from build123d import *

# Parameters (mm, degrees)
F1_DEPTH  = 46
F2_R      = 1
F3_DEPTH  = 1.5
F5_DEPTH  = 40
F6_R      = 1.5
F7_DEPTH  = 1.5
F8_R      = 10
F9_DEPTH  = 1.5
F10_DEPTH = 1.259
F11_DEPTH = 1.259


with BuildPart() as f1:
    # F0 (on Top) → F1 (new body)
    with BuildSketch(Plane.XY):
        Polygon((-20, 74.7819926235), (-21.5, 74.7819926235), (-21.5, 16.0825311363), (-1.5, -0.6994614872), (-1.5, -10), (0, -10), (0, 0), (-20, 16.7819926235), align=None)
    extrude(amount=F1_DEPTH)

    # F2 (on face) → F3 (cut, through all)
    with BuildSketch(Plane(origin=(-1.5, 0, 0), x_dir=(0, -1, 0), z_dir=(-1, 0, 0))):
        with Locations((6, 8)):
            Circle(F2_R)
        with Locations((6, 38)):
            Circle(F2_R)
    extrude(amount=-F3_DEPTH, mode=Mode.SUBTRACT)

    # F4 (on face) → F5 (join)
    with BuildSketch(Plane(origin=(0, 74.7819926235, 0), x_dir=(-1, 0, 0), z_dir=(0, 1, 0))):
        Polygon((0, 58.2678901674), (0, 48.2678901674), (20, 44.7413505532), (21.5, 44.7413505532), (21.5, 46), (1.5, 49.5265396142), (1.5, 58.2678901674), align=None)
        Polygon((21.5, 1.2586494468), (20, 1.2586494468), (0, -2.2678901674), (0, -12.2678901674), (1.5, -12.2678901674), (1.5, -3.5265396142), (21.5, 0), align=None)
    extrude(amount=-F5_DEPTH)

    # F6 (on face) → F7 (cut, through all)
    with BuildSketch(Plane(origin=(-1.5, 0, 0), x_dir=(0, -1, 0), z_dir=(-1, 0, 0))):
        with Locations((-71.9999926235, -8)):
            Circle(F6_R)
        with Locations((-41.9999926235, -8)):
            Circle(F6_R)
        with Locations((-41.9999926235, 54)):
            Circle(F6_R)
        with Locations((-71.9999926235, 54)):
            Circle(F6_R)
    extrude(amount=-F7_DEPTH, mode=Mode.SUBTRACT)

    # F8 (on face) → F9 (cut, through all)
    with BuildSketch(Plane(origin=(-21.5, 0, 0), x_dir=(0, -1, 0), z_dir=(-1, 0, 0))):
        with Locations((-49.7819926235, 23)):
            Circle(F8_R)
    extrude(amount=-F9_DEPTH, mode=Mode.SUBTRACT)

    # F10 (cut): a face of the model
    f10_faces = [f1.faces().sort_by_distance(p)[0] for p in [
        (-10.3193093541, 8.0104582418, 0),
    ]]
    extrude(f10_faces, amount=-F10_DEPTH, mode=Mode.SUBTRACT)

    # F11 (cut): a face of the model
    f11_faces = [f1.faces().sort_by_distance(p)[0] for p in [
        (-10.3193093541, 8.0104582418, 46),
    ]]
    extrude(f11_faces, amount=-F11_DEPTH, mode=Mode.SUBTRACT)


solid = f1.part
Geometry: final body of the model. Coordinates: model frame, mm. A direction names the side the tool comes from. Round coordinates to 2 decimals unless told otherwise and drop trailing zeros. Loops run counter-clockwise (first coordinate to the right, second up) from the corner with the lowest first, then second, coordinate; pieces in that order, holes last. Notation, with made-up numbers: (-18, 5.5) -> (40, 5.5) arc R22 cw to (40, 31.5) -> close; hole circle Ø2 at (-29, 55.25). An arc over 180 degrees is marked (long way). One line per question, with ' | ' between items. Start each with the question number.
1. Section D-D on y = 36. Output: boundary loops of the cut face in (x, z), and give its area (3 significant figures).
2. Section A-A on z = 8. Output: boundary loops of the cut face in (x, y), and give its area (3 significant figures).
3. Line query: line 1 along Z through (x, y) = (-0.85, -6); line 2 along X through (y, z) = (61, 4.5); line 3 along X through (y, z) = (-4, 33). Output: solid intervals per line, ascending. Write a range as [from, to].
4. Section B-B on y = -6. Output: boundary loops of the cut face in (x, z), and give its area (3 significant figures).
5. Contact query for flat-ended pins moving along their axis: pin 1 (2.5 mm diameter, centred on y = 51, z = 55, fed in from -X); pin 2 (2.5 mm diameter, centred on y = 42, z = -8, fed in from -X); pin 3 (8 mm diameter, centred on x = -3.5, y = 0, fed in from +Z); pin 4 (1 mm diameter, centred on x = -4.5, z = 23, fed in from -Y). Output: stop coordinate, or through.
6. Section C-C on z = -8. Output: boundary loops of the cut face in (x, y), and give its area (3 significant figures).
7. Set-up query: faces 5 (the face through (-1.5, 55, 54)), 6 (the face through (-20, 39, 23)), 7 (the face through (-13.2, 10.8, 44.741)). Return all of +Z, -Z, +X, -X, +Y, -Y with unobstructed straight access to the full face (end or side cutting, diameter ignored); none if empty.
8. Mould query, pull axis Y, two halves, no side actions, for faces 1 (the face through (-0.76, 70.614, -8.575)), 2 (the face through (-8, 34.782, -2)), 3 (the face through (-9.86, 8.274, 22.696)), 4 (the face through (-1.5, 55, -8)). Classes: pulls with the +Y half, pulls with the -Y half, needs draft (parallel to the pull), parting line crosses it, or undercut.
Returned:
1) outline: (-21.5, 0) -> (-1.5, -3.53) -> (-1.5, -12.27) -> (0, -12.27) -> (0, -2.27) -> (-20, 1.26) -> (-20, 44.74) -> (0, 48.27) -> (0, 58.27) -> (-1.5, 58.27) -> (-1.5, 49.53) -> (-21.5, 46) -> close | area: 156 mm2
2) outline: (-21.5, 16.08) -> (-1.5, -0.7) -> (-1.5, -5) -> (0, -5) -> (0, 0) -> (-20, 16.78) -> (-20, 74.78) -> (-21.5, 74.78) -> close; (-1.5, -10) -> (0, -10) -> (0, -7) -> (-1.5, -7) -> close | area: 138 mm2
3) line 1: z = [1.26, 7], [9, 37], [39, 44.74] | line 2: x = [-21.5, -20] | line 3: x = [-1.5, 0]
4) outline: (-1.5, 1.26) -> (0, 1.26) -> (0, 7) -> (-1.5, 7) -> close; (-1.5, 9) -> (0, 9) -> (0, 37) -> (-1.5, 37) -> close; (-1.5, 39) -> (0, 39) -> (0, 44.74) -> (-1.5, 44.74) -> close | area: 59.2 mm2
5) pin 1: stops at x = -1.5 | pin 2: passes through | pin 3: stops at z = 44.74 | pin 4: stops at y = 1.4
6) outline: (-1.5, 34.78) -> (0, 34.78) -> (0, 40.5) -> (-1.5, 40.5) -> close; (-1.5, 43.5) -> (0, 43.5) -> (0, 70.5) -> (-1.5, 70.5) -> close; (-1.5, 73.5) -> (0, 73.5) -> (0, 74.78) -> (-1.5, 74.78) -> close | area: 51.0 mm2
7) face 5: +Z, -X, +Y, -Y | face 6: +X, +Y | face 7: +Z, +X, -X, -Y
8) face 1: undercut | face 2: pulls with the -Y half | face 3: pulls with the +Y half | face 4: needs draft
